from build123d import *

# Parameters (mm, degrees)
EXTRUDE1_DEPTH = 19
SKETCH2_R      = 1.5
EXTRUDE5_DEPTH = 8.5
SKETCH3_W      = 0.4
SKETCH3_H      = 15.2
EXTRUDE6_DEPTH = 20.0000001


with BuildPart() as part:
    # Sketch1 → Extrude1 (new body)
    with BuildSketch(Plane.XY):
        with BuildLine():
            Line((0, 4), (0, 7.6))
            Line((0, 7.6), (-7.5, 7.6))
            Line((-7.5, 7.6), (-7.5, -7.6))
            Line((-7.5, -7.6), (0, -7.6))
            Line((0, -7.6), (0, -4))
            ThreePointArc((0, -4), (-4, 0), (0, 4))
        make_face()
    extrude(amount=EXTRUDE1_DEPTH)

    # Sketch2 → Extrude5 (cut, through all)
    with BuildSketch(Plane(origin=(-7.5, 0, 0), x_dir=(0, 0, -1), z_dir=(1, 0, 0))):
        with Locations((-3.175, 4.425)):
            Circle(SKETCH2_R)
        with Locations((-15, 4.425)):
            Circle(SKETCH2_R)
        with Locations((-15, -4.425)):
            Circle(SKETCH2_R)
        with Locations((-3.175, -4.425)):
            Circle(SKETCH2_R)
    extrude(amount=EXTRUDE5_DEPTH, mode=Mode.SUBTRACT)

    # Sketch3 → Extrude6 (cut, through all)
    with BuildSketch(Plane.XY.offset(19)):
        with Locations((-0.2, 0)):
            Rectangle(SKETCH3_W, SKETCH3_H)
    extrude(amount=-EXTRUDE6_DEPTH, mode=Mode.SUBTRACT)


solid = part.part
The model under review builds one solid part; all positions refer to its coordinate system, in mm. Round coordinates to 2 decimals unless told otherwise and drop trailing zeros. Loops run counter-clockwise (first coordinate to the right, second up) from the corner with the lowest first, then second, coordinate; pieces in that order, holes last. Notation, with made-up numbers: (-3.5, 16.5) -> (10.5, 16.5) arc R25 ccw to (10.5, 39.5) -> close; hole circle Ø4 at (54, 83.25). An arc over 180 degrees is marked (long way). Write item = value, one per line. Start each with the question number.
Item 1: Take a section at A-A on z = 15.25. Give the boundary of the cut face in (x, y).
Item 2: Mouldability with a two-part tool opening along Z and no side actions: class faces 1 (the flat face through (-5, 0, 19)), 2 (the cylindrical face through (-4, 5.912, 3.37)), 3 (the flat face through (-0.4, -6, 10)) as released by +Z, released by -Z, zero draft, split by the parting line, or undercut.
Item 3: Take a section at C-C on y = 5. Give the boundary of the cut face in (x, z), plus the area to 3 significant figures.
Item 4: Take a section at B-B on x = -1. Give the boundary of the cut face in (y, z) (3 decimals), plus the area to 3 significant figures.
Item 5: To check wall thickness, follow L1, parallel to Y at x = -5.5, z = 15 (3 decimals); L2, parallel to Y at x = -6.25, z = 16; L3, parallel to Z at x = -1, y = -4.75. State the ranges of each line that lie inside material, in increasing order.
Item 6: Insertion check: pin 1 (1 mm diameter, centred on x = -3, y = 3.5, fed in from -Z); pin 2 (2.5 mm diameter, centred on y = 4.425, z = 3.175, fed in from +X). Each pin has a flat end and moves straight along its axis. Give the tip position at first contact, or say it passes through.
Item 7: Take a section at D-D on x = -4.75. Give the boundary of the cut face in (y, z) (3 decimals).
Result:
q1.outline = (-7.5, -7.6) -> (-0.4, -7.6) -> (-0.4, -5.9) -> (-7.5, -5.9) -> close; (-7.5, -2.95) -> (-2.71, -2.95) arc R4 cw to (-2.71, 2.95) -> (-7.5, 2.95) -> close; (-7.5, 5.9) -> (-0.4, 5.9) -> (-0.4, 7.6) -> (-7.5, 7.6) -> close
q2.face_1 = released by +Z
q2.face_2 = undercut
q2.face_3 = zero draft
q3.outline = (-7.5, 0) -> (-0.4, 0) -> (-0.4, 1.79) -> (-7.5, 1.79) -> close; (-7.5, 4.56) -> (-0.4, 4.56) -> (-0.4, 13.61) -> (-7.5, 13.61) -> close; (-7.5, 16.39) -> (-0.4, 16.39) -> (-0.4, 19) -> (-7.5, 19) -> close
q3.area = 95.6 mm²
q4.outline = (-7.6, 0) -> (-3.873, 0) -> (-3.873, 1.78) arc R1.5 cw (long way) to (-3.873, 4.57) -> (-3.873, 13.605) arc R1.5 cw (long way) to (-3.873, 16.395) -> (-3.873, 19) -> (-7.6, 19) -> close; (3.873, 0) -> (7.6, 0) -> (7.6, 19) -> (3.873, 19) -> (3.873, 16.395) arc R1.5 cw (long way) to (3.873, 13.605) -> (3.873, 4.57) arc R1.5 cw (long way) to (3.873, 1.78) -> close
q4.area = 121 mm²
q5.L1 = -7.6 to -5.925, -2.925 to 2.925, 5.925 to 7.6
q5.L2 = -7.6 to -5.54, -3.31 to 3.31, 5.54 to 7.6
q5.L3 = 0 to 1.71, 4.64 to 13.54, 16.46 to 19
q6.pin_1 = 0
q6.pin_2 = through
q7.outline = (-7.6, 0) -> (7.6, 0) -> (7.6, 19) -> (-7.6, 19) -> close; hole circle Ø3 at (-4.425, 3.175); hole circle Ø3 at (-4.425, 15); hole circle Ø3 at (4.425, 3.175); hole circle Ø3 at (4.425, 15)
